Verification items for the finished model (mm, model axes). A direction names the side the tool comes from. Round coordinates to 2 decimals unless told otherwise and drop trailing zeros. Write each loop counter-clockwise with the first axis right and the second up, starting at its lowest first coordinate (ties: lowest second). Pieces come first, ordered by that corner, then holes. Notation, with made-up numbers: (6.25, 54) - (65.25, 54) arc R16 ccw to (65.25, 65) - close; hole circle Ø1 at (-21, 62). An arc over 180 degrees is marked (long way). Answer as a JSON object with one key per item and string values.
```python
from build123d import *

# Parameters (mm, degrees)
BOSS_EXTRUDE1_DEPTH       = 55
SHELL1_T                  = -2
BOSS_EXTRUDE2_DEPTH       = 10
M3X0_5_TAPPED_HOLE1_D     = 2.5
M3X0_5_TAPPED_HOLE1_DEPTH = 7.5
M3X0_5_TAPPED_HOLE1_TIP   = 0.751075774
BOSS_EXTRUDE3_REACH       = 69.127
SKETCH5_W                 = 66
SKETCH5_H                 = 2
SKETCH6_W                 = 40
SKETCH6_H                 = 15
CUT_EXTRUDE1_DEPTH        = 10
F_3_0MM_DOWEL_HOLE1_D     = 3
F_3_0MM_DOWEL_HOLE1_DEPTH = 4
F_3_0MM_DOWEL_HOLE1_TIP   = 0.901290929
SKETCH9_W                 = 20
SKETCH9_H                 = 16
CUT_EXTRUDE2_DEPTH        = 2
FILLET1_R                 = 2


with BuildPart() as part:
    # Sketch1 → Boss-Extrude1 (new body)
    with BuildSketch(Plane.XY):
        with BuildLine():
            Line((-15, 16), (15, 16))
            ThreePointArc((15, 16), (29.142135624, 10.142135624), (35, -4))
            Line((35, -4), (35, -6))
            ThreePointArc((35, -6), (32.071067812, -13.071067812), (25, -16))
            Line((25, -16), (-25, -16))
            ThreePointArc((-25, -16), (-32.071067812, -13.071067812), (-35, -6))
            Line((-35, -6), (-35, -4))
            ThreePointArc((-35, -4), (-29.142135624, 10.142135624), (-15, 16))
        make_face()
    extrude(amount=BOSS_EXTRUDE1_DEPTH)

    # Shell1
    shell1_openings = [part.faces().sort_by_distance(p)[0] for p in [
        (0, -0.685833175, 0),
    ]]
    offset(amount=SHELL1_T, openings=shell1_openings, kind=Kind.INTERSECTION)

    # Sketch2 → Boss-Extrude2 (add)
    with BuildSketch(Plane(origin=(0, 0, 0), x_dir=(-1, 0, 0), z_dir=(0, 0, -1))):
        with BuildLine():
            Line((-15, 4.48), (-30.87732975, 4.48))
            ThreePointArc((-30.87732975, 4.48), (-24.256349172, 11.437616396), (-15, 14))
            Line((-15, 14), (-15, 4.48))
        make_face()
        with BuildLine():
            Line((15, 4.48), (15, 14))
            ThreePointArc((15, 14), (24.256349172, 11.437616396), (30.87732975, 4.48))
            Line((30.87732975, 4.48), (15, 4.48))
        make_face()
    extrude(amount=-BOSS_EXTRUDE2_DEPTH)

    # M3x0.5 Tapped Hole1
    with Locations(Plane(origin=(0, 0, 0), x_dir=(-1, 0, 0), z_dir=(0, 0, -1))):
        with Locations((-18.4, 8), (21.6, 8)):
            Hole(M3X0_5_TAPPED_HOLE1_D / 2, depth=M3X0_5_TAPPED_HOLE1_DEPTH)
            with Locations((0, 0, -(M3X0_5_TAPPED_HOLE1_DEPTH + M3X0_5_TAPPED_HOLE1_TIP / 2))):  # 118° drill point
                Cone(0, M3X0_5_TAPPED_HOLE1_D / 2, M3X0_5_TAPPED_HOLE1_TIP, mode=Mode.SUBTRACT)

    # Sketch5 → Boss-Extrude3 (add, up to next)
    with BuildSketch(Plane(origin=(0, 0, 0), x_dir=(-1, 0, 0), z_dir=(0, 0, -1)), mode=Mode.PRIVATE) as boss_extrude3_sk1:
        with Locations((0, -6.52)):
            Rectangle(SKETCH5_W, SKETCH5_H)
    boss_extrude3_tool1 = extrude(boss_extrude3_sk1.sketch, amount=-BOSS_EXTRUDE3_REACH, mode=Mode.PRIVATE) - part.part
    add(boss_extrude3_tool1.solids().sort_by_distance((0, -6.52, 0))[0])

    # Sketch6 → Cut-Extrude1 (cut)
    with BuildSketch(Plane(origin=(0, 0, 53), x_dir=(-1, 0, 0), z_dir=(0, 0, -1))):
        with Locations((0, 1.98)):
            Rectangle(SKETCH6_W, SKETCH6_H)
    extrude(amount=-CUT_EXTRUDE1_DEPTH, mode=Mode.SUBTRACT)

    # Ø3.0mm Dowel Hole1
    with Locations(Plane(origin=(0, -5.52, 0), x_dir=(1, 0, 0), z_dir=(0, 1, 0))):
        with Locations((-17, -47), (-17, -22), (17, -34.5)):
            Hole(F_3_0MM_DOWEL_HOLE1_D / 2, depth=F_3_0MM_DOWEL_HOLE1_DEPTH)
            with Locations((0, 0, -(F_3_0MM_DOWEL_HOLE1_DEPTH + F_3_0MM_DOWEL_HOLE1_TIP / 2))):  # 118° drill point
                Cone(0, F_3_0MM_DOWEL_HOLE1_D / 2, F_3_0MM_DOWEL_HOLE1_TIP, mode=Mode.SUBTRACT)

    # Sketch9 → Cut-Extrude2 (cut)
    with BuildSketch(Plane(origin=(0, -5.52, 0), x_dir=(1, 0, 0), z_dir=(0, 1, 0))):
        with Locations((-23, -34.5)):
            Rectangle(SKETCH9_W, SKETCH9_H)
    extrude(amount=-CUT_EXTRUDE2_DEPTH, mode=Mode.SUBTRACT)

    # Fillet1
    fillet1_edges = [part.edges().sort_by_distance(p)[0] for p in [
        (29.142135624, 10.142135624, 55),
        (0, 16, 55),
        (-29.142135624, 10.142135624, 55),
        (-35, -5, 55),
        (-32.071067812, -13.071067812, 55),
        (0, -16, 55),
        (32.071067812, -13.071067812, 55),
        (35, -5, 55),
    ]]
    fillet(fillet1_edges, radius=FILLET1_R)


solid = part.part
```
Q1. Gauge pin test, flat ends, axial feed: P1, Ø1, axis at y = 11, z = 21, coming from the +X side (3 decimals); P2, Ø6, axis at y = 7.5, z = 21, coming from the +X side; P3, Ø1.5, axis at y = -12, z = 21, coming from the +X side. Record the tip position at first contact, or that the pin passes through.
Geometry check:
{"P1": "stops at x = 28.775", "P2": "stops at x = 33.1", "P3": "stops at x = 33.51"}
Q2. Section check A-A, the plane x = -1. Record the cut outline in (y, z).
Geometry check:
{"outline": "(-16, 0) - (-14, 0) - (-14, 53) - (-7.52, 53) - (-7.52, 0) - (-5.52, 0) - (-5.52, 55) - (-14, 55) arc R2 ccw to (-16, 53) - close; (9.48, 53) - (14, 53) - (14, 0) - (16, 0) - (16, 53) arc R2 ccw to (14, 55) - (9.48, 55) - close"}
Q3. Release check for a two-part mould opening along Z. For faces 1 (the cylindrical face through (-21.87, 6.78, 3.8)), 2 (the flat face through (0, -11, 53)), 3 (the flat face through (-23, -7, 42.5)) record: released by +Z, released by -Z, zero draft, split by the parting line, or undercut.
Geometry check:
{"face 1": "zero draft", "face 2": "released by -Z", "face 3": "undercut"}
Q4. Section check C-C, the plane z = 47. Record the cut outline in (x, y).
Geometry check:
{"outline": "(-35, -6) arc R10 ccw to (-25, -16) - (25, -16) arc R10 ccw to (35, -6) - (35, -4) arc R20 ccw to (15, 16) - (-15, 16) arc R20 ccw to (-35, -4) - close; hole (-33, -5.52) - (-18.5, -5.52) - (-18.5, -7.52) - (-32.85, -7.52) arc R8 ccw to (-25, -14) - (25, -14) arc R8 ccw to (32.85, -7.52) - (-15.5, -7.52) - (-15.5, -5.52) - (33, -5.52) - (33, -4) arc R18 ccw to (15, 14) - (-15, 14) arc R18 ccw to (-33, -4) - close"}
Q5. Material ranges on line 1 along Z through (x, y) = (-17, -6); line 2 along Y through (x, z) = (-13, 14); line 3 along X through (y, z) = (8, 2.5), recorded low to high. Write a range as [from, to].
Geometry check:
{"line 1": "z = [0, 20.5], [23.5, 26.5], [42.5, 45.5], [48.5, 55]", "line 2": "y = [-16, -14], [-7.52, -5.52], [14, 16]", "line 3": "x = [-31, -22.85], [-20.35, -15], [15, 17.15], [19.65, 31]"}
Q6. Section check D-D, the plane z = 28. Record the cut outline in (x, y), then the cut area to 3 significant figures.
Geometry check:
{"outline": "(-35, -6) arc R10 ccw to (-25, -16) - (25, -16) arc R10 ccw to (35, -6) - (35, -4) arc R20 ccw to (15, 16) - (-15, 16) arc R20 ccw to (-35, -4) - close; hole (-33, -7.52) - (-32.85, -7.52) arc R8 ccw to (-25, -14) - (25, -14) arc R8 ccw to (32.85, -7.52) - (-13, -7.52) - (-13, -5.52) - (33, -5.52) - (33, -4) arc R18 ccw to (15, 14) - (-15, 14) arc R18 ccw to (-33, -4) - close", "area": "436 mm2"}
Q7. Set-up check for faces 4 (the flat face through (15, 9, 5)), 5 (the cylindrical face through (34.43, -5.01, 54.4)), 6 (the cylindrical face through (-15.89, -6.53, 20.99)): record each of +Z, -Z, +X, -X, +Y, -Y from which the full face is reachable in a straight line by a thin tool's end or side.
Geometry check:
{"face 4": "-Z", "face 5": "+Z, +X, +Y, -Y", "face 6": "none"}
Q8. Section check B-B, the plane z = 11. Record the cut outline in (x, y).
Geometry check:
{"outline": "(-35, -6) arc R10 ccw to (-25, -16) - (25, -16) arc R10 ccw to (35, -6) - (35, -4) arc R20 ccw to (15, 16) - (-15, 16) arc R20 ccw to (-35, -4) - close; hole (-33, -5.52) - (33, -5.52) - (33, -4) arc R18 ccw to (15, 14) - (-15, 14) arc R18 ccw to (-33, -4) - close; hole (-32.85, -7.52) arc R8 ccw to (-25, -14) - (25, -14) arc R8 ccw to (32.85, -7.52) - close"}
